from build123d import *

# Parameters (mm, degrees)
SKETCH1_R                          = 34.798
SKETCH1_R_2                        = 32.258
BOSS_EXTRUDE1_DEPTH                = 11.684
F_3_16_0_1875_DIAMETER_HOLE1_D     = 4.7625
F_3_16_0_1875_DIAMETER_HOLE1_DEPTH = 54.102
F_3_16_0_1875_DIAMETER_HOLE1_TIP   = 1.430799349
SKETCH3_R                          = 33.274
SKETCH3_R_2                        = 32.258
CUT_EXTRUDE1_DEPTH                 = 6.604


with BuildPart() as part:
    # Sketch1 → Boss-Extrude1 (new body)
    with BuildSketch(Plane.XY):
        Circle(SKETCH1_R)
        Circle(SKETCH1_R_2, mode=Mode.SUBTRACT)
    extrude(amount=BOSS_EXTRUDE1_DEPTH)

    # 3/16 (0.1875) Diameter Hole1
    with Locations(Plane(origin=(34.798, 0, 2.54), x_dir=(0, 1, 0), z_dir=(1, 0, 0))):
        with Locations((0, 0)):
            Hole(F_3_16_0_1875_DIAMETER_HOLE1_D / 2, depth=F_3_16_0_1875_DIAMETER_HOLE1_DEPTH)
            with Locations((0, 0, -(F_3_16_0_1875_DIAMETER_HOLE1_DEPTH + F_3_16_0_1875_DIAMETER_HOLE1_TIP / 2))):  # 118° drill point
                Cone(0, F_3_16_0_1875_DIAMETER_HOLE1_D / 2, F_3_16_0_1875_DIAMETER_HOLE1_TIP, mode=Mode.SUBTRACT)

    # Sketch3 → Cut-Extrude1 (cut)
    with BuildSketch(Plane(origin=(0, 0, 0), x_dir=(-1, 0, 0), z_dir=(0, 0, -1))):
        Circle(SKETCH3_R)
        Circle(SKETCH3_R_2, mode=Mode.SUBTRACT)
    extrude(amount=-CUT_EXTRUDE1_DEPTH, mode=Mode.SUBTRACT)


solid = part.part
The listing builds one solid part. Answer for the finished solid, in the listing's coordinates (mm). A direction names the side the tool comes from. Round coordinates to 2 decimals unless told otherwise and drop trailing zeros. Order: outer loops, then holes, each group sorted by start corner. A loop starts at its lowest first (then second) coordinate and runs counter-clockwise, first axis right, second up. Notation, with made-up numbers: (39.5, -17.75) - (76.5, -17.75) arc R16 ccw to (76.5, -10.75) - close; hole circle Ø8 at (-23, 28). An arc over 180 degrees is marked (long way). Write item = value, one per line. Start each with the question number.
1) For faces 1 (the cylindrical face through (-31.74, 9.99, 3.26)), 2 (the cylindrical face through (30.77, 9.69, 9.11)), determine the directions among +Z, -Z, +X, -X, +Y, -Y from which every point of the face is accessible in a straight line to the end or side of a thin tool.
2) Straight lines are drawn through the part: L1, parallel to Z at x = 33.5, y = 0; L2, parallel to Y at x = 0, z = 9.15; L3, parallel to X at y = -1, z = 5.25. For each, find the intervals that lie inside material, in ascending order.
3) For a pull along Y with two mould halves and no side action, classify faces 3 (the flat face through (10, -31, 11.684)), 4 (the cylindrical face through (-7.54, -33.97, 5.76)), 5 (the cylindrical face through (33.98, -2.27, 3.26)) as released by +Y, released by -Y, zero draft, split by the parting line, or undercut.
4) Given pin 1 (12 mm diameter, centred on x = 25.5, y = 27.5, fed in from -Z); pin 2 (1.5 mm diameter, centred on x = -17, z = 6.5, fed in from -Y); pin 3 (1 mm diameter, centred on y = 19, z = 8.5, fed in from -X); pin 4 (3 mm diameter, centred on y = -18.5, z = 2.5, fed in from +X), each flat-ended and moving along its own axis, determine where each tip first touches the part or whether it passes through.
5) Section A-A, the plane y = 0 is taken. Write down the section's boundary in (x, z).
6) Section D-D, the plane z = 9.5 is taken. Write down the section's boundary in (x, y).
7) Section B-B, the plane x = 0 is taken. Write down the section's boundary in (y, z), plus the area to 3 significant figures.
8) Section C-C, the plane y = -21 is taken. Write down the section's boundary in (x, z).
Results list:
q1.face_1 = -Z
q1.face_2 = +Z, -Z
q2.L1 = 0 to 0.16, 4.92 to 11.68
q2.L2 = -34.8 to -32.26, 32.26 to 34.8
q2.L3 = -34.78 to -33.26, 33.26 to 34.78
q3.face_3 = zero draft
q3.face_4 = split by the parting line
q3.face_5 = undercut
q4.pin_1 = 0
q4.pin_2 = -30.77
q4.pin_3 = -29.47
q4.pin_4 = 30.36
q5.outline = (-34.8, 0) - (-33.27, 0) - (-33.27, 6.6) - (-32.26, 6.6) - (-32.26, 11.68) - (-34.8, 11.68) - close; (32.26, 6.6) - (33.27, 6.6) - (33.27, 4.92) - (34.8, 4.92) - (34.8, 11.68) - (32.26, 11.68) - close; (33.27, 0) - (34.8, 0) - (34.8, 0.16) - (33.27, 0.16) - close
q6.outline = circle Ø69.6 at (0, 0); hole circle Ø64.52 at (0, 0)
q7.outline = (-34.8, 0) - (-33.27, 0) - (-33.27, 6.6) - (-32.26, 6.6) - (-32.26, 11.68) - (-34.8, 11.68) - close; (32.26, 6.6) - (33.27, 6.6) - (33.27, 0) - (34.8, 0) - (34.8, 11.68) - (32.26, 11.68) - close
q7.area = 45.9 mm^2
q8.outline = (-27.75, 0) - (-25.81, 0) - (-25.81, 6.6) - (-24.49, 6.6) - (-24.49, 11.68) - (-27.75, 11.68) - close; (24.49, 6.6) - (25.81, 6.6) - (25.81, 0) - (27.75, 0) - (27.75, 11.68) - (24.49, 11.68) - close
